Answer from the drawing. Dimensions are ordinates in mm from the lowest x, y and z of the part. Coordinates: 2 decimals unless noted, no trailing zeros. Write each loop counter-clockwise with the first axis right and the second up, starting at its lowest first coordinate (ties: lowest second). Pieces come first, ordered by that corner, then holes.
(1) Determine the mould class of the marked faces 1, 2 and 3 for opening direction X: pulls with the +X half, pulls with the -X half, needs draft (parallel to the pull), parting line crosses it, or undercut.
(2) The part is cut by section B-B, the plane z = 40. Determine the outline of the cut face in (x, y) (1 decimal), and give its area (3 significant figures).
(3) The part is cut by section D-D, the plane x = 49. Determine the outline of the cut face in (y, z).
(4) The part is cut by section C-C, the plane y = 28.5. State how many separate pieces and enclosed holes the cut face has, and give its area (3 significant figures).
(5) Given pin 1 (1.5 mm diameter, centred on y = 32.5, z = 6, fed in from -X); pin 2 (16 mm diameter, centred on x = 75, z = 29, fed in from -Y); pin 3 (3 mm diameter, centred on y = 43.5, z = 45.5, fed in from +X); pin 4 (3 mm diameter, centred on x = 18.5, z = 41, fed in from -Y), each flat-ended and moving along its own axis, determine where each tip first touches the part or whether it passes through.
(6) Straight lines are drawn through the part: line 1 along X through (y, z) = (27, 16) (1 decimal); line 2 along X through (y, z) = (45.5, 20) (1 decimal); line 3 along Y through (x, z) = (76, 10.5). For each, find the intervals that lie inside material, in ascending order.
(7) The part is cut by section A-A, the plane x = 36.5. Determine the outline of the cut face in (y, z), and give its area (3 significant figures).
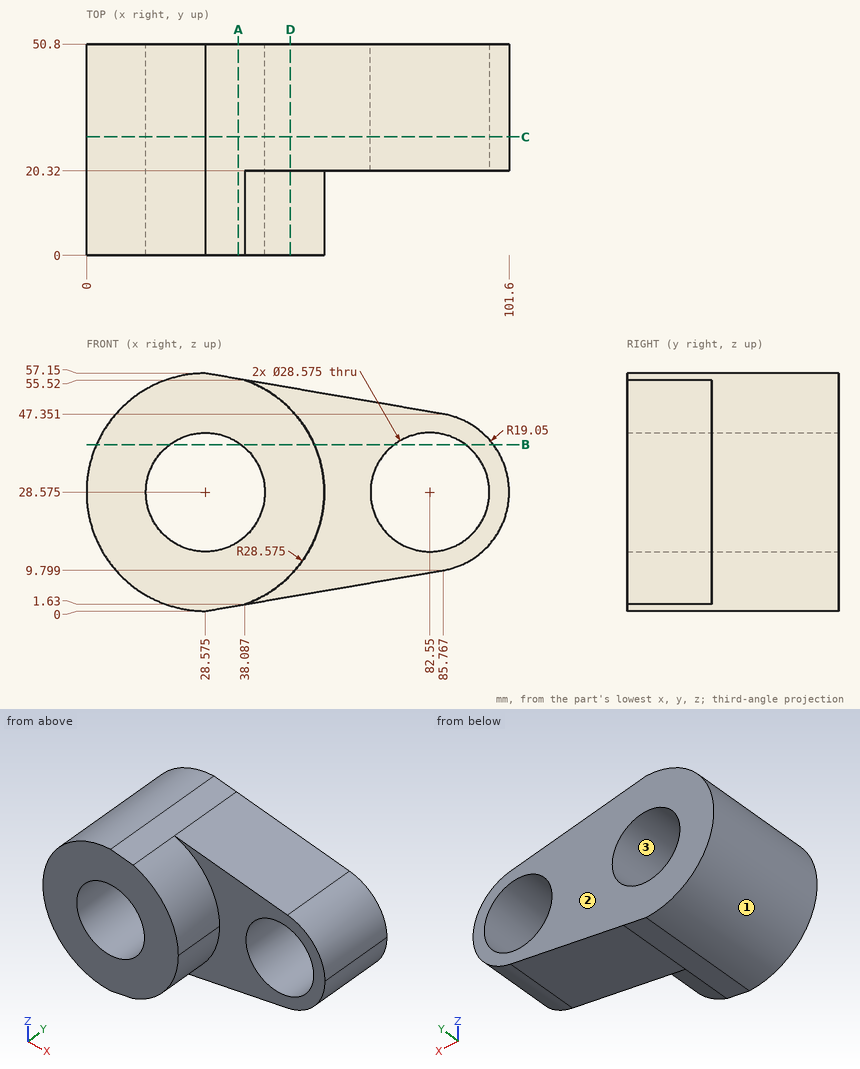
Computed:
1. face 1: pulls with the -X half
1. face 2: needs draft
1. face 3: undercut
2. outline: (2.4, 0) - (20, 0) - (20, 50.8) - (2.4, 50.8) - close; (37.2, 0) - (54.8, 0) - (54.8, 20.3) - (74, 20.3) - (74, 50.8) - (37.2, 50.8) - close; (91.1, 20.3) - (97.8, 20.3) - (97.8, 50.8) - (91.1, 50.8) - close
2. area: 2,580 mm2
3. outline: (0, 8.59) - (20.32, 8.59) - (20.32, 3.5) - (50.8, 3.5) - (50.8, 53.65) - (20.32, 53.65) - (20.32, 48.56) - (0, 48.56) - close
4. separate pieces: 1
4. enclosed holes: 2
4. area: 3,160 mm2
5. pin 1: stops at x = 10.13
5. pin 2: stops at y = 20.32
5. pin 3: stops at x = 93.73
5. pin 4: stops at y = 0
6. line 1: x = 2.9 to 21.8, 35.4 to 75.8, 89.3 to 96.9
6. line 2: x = 1.3 to 17.1, 40 to 71.1, 94 to 99.6
6. line 3: y = 20.32 to 50.8
7. outline: (0, 1.36) - (50.8, 1.36) - (50.8, 16.69) - (0, 16.69) - close; (0, 40.46) - (50.8, 40.46) - (50.8, 55.79) - (0, 55.79) - close
7. area: 1,560 mm2
